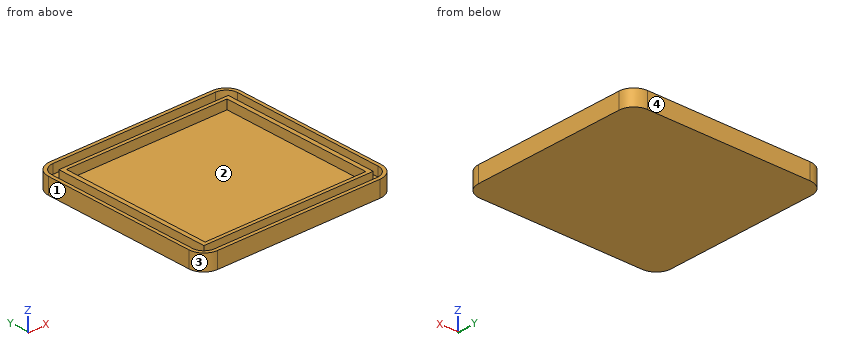
```python
from build123d import *

# Parameters (mm, degrees)
F0_W     = 74
F0_H     = 69.2229812741
F0_W_2   = 70.2229812741
F0_H_2   = 66.2229812741
F1_DEPTH = 3
F2_DEPTH = 7
F3_DEPTH = 7


with BuildPart() as f1:
    # F0 (on Top) → F1 (new body)
    with BuildSketch(Plane.XY):
        with BuildLine():
            Line((42, -33.0089111648), (42, 33.9910888352))
            ThreePointArc((42, 33.9910888352), (40.0961940777, 38.587282913), (35.5, 40.4910888352))
            Line((35.5, 40.4910888352), (-35.5, 40.4910888352))
            ThreePointArc((-35.5, 40.4910888352), (-40.4434463233, 38.4434463233), (-42.4910888352, 33.5))
            Line((-42.4910888352, 33.5), (-42.4910888352, -33.5))
            ThreePointArc((-42.4910888352, -33.5), (-40.587282913, -38.0961940777), (-35.9910888352, -40))
            Line((-35.9910888352, -40), (35.0089111648, -40))
            ThreePointArc((35.0089111648, -40), (39.952357488, -37.952357488), (42, -33.0089111648))
        make_face()
        with BuildLine():
            ThreePointArc((-40.9910888352, 33.5), (-39.3827861515, 37.3827861515), (-35.5, 38.9910888352))
            Line((-35.5, 38.9910888352), (35.5, 38.9910888352))
            ThreePointArc((35.5, 38.9910888352), (39.0355339059, 37.5266227412), (40.5, 33.9910888352))
            Line((40.5, 33.9910888352), (40.5, -33.0089111648))
            ThreePointArc((40.5, -33.0089111648), (38.8916973163, -36.8916973163), (35.0089111648, -38.5))
            Line((35.0089111648, -38.5), (-35.9910888352, -38.5))
            ThreePointArc((-35.9910888352, -38.5), (-39.5266227412, -37.0355339059), (-40.9910888352, -33.5))
            Line((-40.9910888352, -33.5), (-40.9910888352, 33.5))
        make_face(mode=Mode.SUBTRACT)
        with BuildLine():
            Line((35.5, 38.9910888352), (-35.5, 38.9910888352))
            ThreePointArc((-35.5, 38.9910888352), (-39.3827861515, 37.3827861515), (-40.9910888352, 33.5))
            Line((-40.9910888352, 33.5), (-40.9910888352, -33.5))
            ThreePointArc((-40.9910888352, -33.5), (-39.5266227412, -37.0355339059), (-35.9910888352, -38.5))
            Line((-35.9910888352, -38.5), (35.0089111648, -38.5))
            ThreePointArc((35.0089111648, -38.5), (38.8916973163, -36.8916973163), (40.5, -33.0089111648))
            Line((40.5, -33.0089111648), (40.5, 33.9910888352))
            ThreePointArc((40.5, 33.9910888352), (39.0355339059, 37.5266227412), (35.5, 38.9910888352))
        make_face()
        Rectangle(F0_W, F0_H, mode=Mode.SUBTRACT)
        Rectangle(F0_W, F0_H)
        Rectangle(F0_W_2, F0_H_2, mode=Mode.SUBTRACT)
        Rectangle(F0_W_2, F0_H_2)
    extrude(amount=F1_DEPTH)

    # F0 (on Top) → F2 (join)
    with BuildSketch(Plane.XY):
        with BuildLine():
            Line((42, -33.0089111648), (42, 33.9910888352))
            ThreePointArc((42, 33.9910888352), (40.0961940777, 38.587282913), (35.5, 40.4910888352))
            Line((35.5, 40.4910888352), (-35.5, 40.4910888352))
            ThreePointArc((-35.5, 40.4910888352), (-40.4434463233, 38.4434463233), (-42.4910888352, 33.5))
            Line((-42.4910888352, 33.5), (-42.4910888352, -33.5))
            ThreePointArc((-42.4910888352, -33.5), (-40.587282913, -38.0961940777), (-35.9910888352, -40))
            Line((-35.9910888352, -40), (35.0089111648, -40))
            ThreePointArc((35.0089111648, -40), (39.952357488, -37.952357488), (42, -33.0089111648))
        make_face()
        with BuildLine():
            ThreePointArc((-40.9910888352, 33.5), (-39.3827861515, 37.3827861515), (-35.5, 38.9910888352))
            Line((-35.5, 38.9910888352), (35.5, 38.9910888352))
            ThreePointArc((35.5, 38.9910888352), (39.0355339059, 37.5266227412), (40.5, 33.9910888352))
            Line((40.5, 33.9910888352), (40.5, -33.0089111648))
            ThreePointArc((40.5, -33.0089111648), (38.8916973163, -36.8916973163), (35.0089111648, -38.5))
            Line((35.0089111648, -38.5), (-35.9910888352, -38.5))
            ThreePointArc((-35.9910888352, -38.5), (-39.5266227412, -37.0355339059), (-40.9910888352, -33.5))
            Line((-40.9910888352, -33.5), (-40.9910888352, 33.5))
        make_face(mode=Mode.SUBTRACT)
    extrude(amount=F2_DEPTH)

    # F0 (on Top) → F3 (join)
    with BuildSketch(Plane.XY):
        Rectangle(F0_W, F0_H)
        Rectangle(F0_W_2, F0_H_2, mode=Mode.SUBTRACT)
    extrude(amount=F3_DEPTH)


solid = f1.part
```
Geometry check sheet. Reference: the model listing, model coordinates, mm. Face numbers are marked on the shaded views. Give positions to 0.01 mm unless a question says otherwise; leave off trailing zeros. Order: outer loops, then holes, each group sorted by start corner. A loop starts at its lowest first (then second) coordinate and runs counter-clockwise, first axis right, second up.
1. Section check A-A, the plane z = 5. Enter the section's corners in (x, y), and give its area (3 significant figures).
2. Section check C-C, the plane x = -15. Enter the section's corners in (y, z).
3. Release check for a two-part mould opening along Y. For the marked faces 1, 2, 3 and 4 record: pulls with the +Y half, pulls with the -Y half, needs draft (parallel to the pull), parting line crosses it, or undercut.
4. Gauge pin test, flat end, axial feed: pin 1 Ø1 at (x, y) = (-1, 13.5) entering from +Z. Record the tip position at first contact, or that the pin passes through.
5. Section check B-B, the plane y = -3.5. Enter the section's corners in (x, z), and give its area (3 significant figures).
6. Thickness scan on L1, parallel to Y at x = 28, z = 5; L2, parallel to X at y = -15, z = 4; L3, parallel to Z at x = -25, y = -24.5. Record the ranges inside material, lowest first.
Values follow:
1. outline: (-42.49, -33.5) arc R6.5 ccw to (-35.99, -40) - (35.01, -40) arc R6.99 ccw to (42, -33.01) - (42, 33.99) arc R6.5 ccw to (35.5, 40.49) - (-35.5, 40.49) arc R6.99 ccw to (-42.49, 33.5) - close; (-37, -34.61) - (37, -34.61) - (37, 34.61) - (-37, 34.61) - close; hole (-40.99, -33.5) arc R5 ccw to (-35.99, -38.5) - (35.01, -38.5) arc R5.49 ccw to (40.5, -33.01) - (40.5, 33.99) arc R5 ccw to (35.5, 38.99) - (-35.5, 38.99) arc R5.49 ccw to (-40.99, 33.5) - close; hole (-35.11, -33.11) - (35.11, -33.11) - (35.11, 33.11) - (-35.11, 33.11) - close
1. area: 943 mm2
2. outline: (-40, 0) - (40.49, 0) - (40.49, 7) - (38.99, 7) - (38.99, 3) - (34.61, 3) - (34.61, 7) - (33.11, 7) - (33.11, 3) - (-33.11, 3) - (-33.11, 7) - (-34.61, 7) - (-34.61, 3) - (-38.5, 3) - (-38.5, 7) - (-40, 7) - close
3. face 1: needs draft
3. face 2: undercut
3. face 3: pulls with the -Y half
3. face 4: pulls with the +Y half
4. pin 1: stops at z = 3
5. outline: (-42.49, 0) - (42, 0) - (42, 7) - (40.5, 7) - (40.5, 3) - (37, 3) - (37, 7) - (35.11, 7) - (35.11, 3) - (-35.11, 3) - (-35.11, 7) - (-37, 7) - (-37, 3) - (-40.99, 3) - (-40.99, 7) - (-42.49, 7) - close
5. area: 281 mm2
6. L1: y = -40 to -38.5, -34.61 to -33.11, 33.11 to 34.61, 38.99 to 40.49
6. L2: x = -42.49 to -40.99, -37 to -35.11, 35.11 to 37, 40.5 to 42
6. L3: z = 0 to 3
